Solid Edge part; units mm, degrees
sketch "Sketch1" plane through (0, 0, 0) normal (0, -1, 0) x (1, 0, 0)
  line L0 (0, 21.7) -> (4.505, 21.7)
  line L1 (4.505, 21.7) -> (4.505, 18.25)
  line L2 (4.505, 18.25) -> (2.1, 18.25)
  line L3 (2.1, 18.25) -> (2.1, 17.85)
  line L4 (2.1, 17.85) -> (2.5, 17.85)
  line L5 (2.5, 17.85) -> (2.5, 7.25)
  line L6 (2.5, 7.25) -> (2, 7.25)
  line L7 (2, 7.25) -> (2, 0)
  line L8 (2, 0) -> (0, 0)
  dimension "D1" = 4.505
  dimension "D2" = 2.1
  dimension "D3" = 2
  dimension "D4" = 2.5
  dimension "D5" = 2
revolve "RevolvedProtrusion1" add sketch "Sketch1" angle 360 about axis through (0, 0, 0) along (0, 0, 1)
chamfer "Chamfer1" distance 0.3 angle 45 3 edges at (-2.5, 0, 17.85) (-4.505, 0, 21.7) (-2, 0, 0)
fillet "Round_1" radius 0.2 4 edges at (-4.505, 0, 18.25) (-2.1, 0, 18.25) (-2.5, 0, 7.25) (-2.5, 0, 17.55)
sketch "Sketch2" plane through (0, 0, 21.7) normal (0, 0, 1) x (1, 0, 0)
  line L0 (1.5, 0.866) -> (0, 1.7321)
  line L1 (0, 1.7321) -> (-1.5, 0.866)
  line L2 (-1.5, 0.866) -> (-1.5, -0.866)
  line L3 (-1.5, -0.866) -> (0, -1.7321)
  line L4 (0, -1.7321) -> (1.5, -0.866)
  line L5 (1.5, -0.866) -> (1.5, 0.866)
extrude "ExtrudedCutout_1" cut sketch "Sketch2" against normal blind 2.4
properties material "Stainless Steel, 304"
Verification items for the finished model (mm, model axes). A direction names the side the tool comes from. Coordinates: 2 decimals unless noted, no trailing zeros. Order: outer loops, then holes, each group sorted by start corner. A loop starts at its lowest first (then second) coordinate and runs counter-clockwise, first axis right, second up. Notation, with made-up numbers: (-17, 18.25) -> (17, 18.25) arc R31 cw to (17, 51.25) -> close; hole circle Ø10 at (-3.5, 26). An arc over 180 degrees is marked (long way). Put each result on its own line as item: value. Start each with the question number.
1. Access from +Z, -Z, +X, -X, +Y, -Y to the whole of each face (thin tool, end or side, straight path). Record for faces 5 (the flat face through (0.74, -1.305, 20.517)), 6 (the flat face through (0, 0, 0)), 7 (the cylindrical face through (0, 2, 4)).
2. Go/stop test with flat-tipped pins: pin 1 Ø1 at (y, z) = (2.5, 13) entering from -X; pin 2 Ø2 at (y, z) = (0.5, 10.5) entering from -X; pin 3 Ø1.5 at (y, z) = (-0.5, 12.5) entering from +X. Record where each tip stops, or that it passes through.
3. Cross-section at B-B, the plane z = 4.5. Record the boundary of the cut face in (x, y).
4. Cross-section at A-A, the plane z = 8.75. Record the boundary of the cut face in (x, y), then the cut area to 3 significant figures.
5. Material ranges on L1, parallel to X at y = 2, z = 9.25; L2, parallel to Z at x = 3.75, y = -0.25; L3, parallel to Y at x = -1, z = 1.5, recorded low to high. Write a range as [from, to].
6. Mould release check, pull along Y, two halves, no side actions. Record for faces 1 (the flat face through (2, 0, 21.7)), 2 (the cylindrical face through (4.3, -1.35, 19.9)), 3 (the flat face through (0, 0, 19.3)), 4 (the flat face through (-0.74, 1.305, 20.517)): released by +Y, released by -Y, zero draft, split by the parting line, or undercut.
Computed:
1. face 5: +Z
1. face 6: -Z, +X, -X, +Y, -Y
1. face 7: -Z
2. pin 1: x = -1.5
2. pin 2: x = -2.5
2. pin 3: x = 2.5
3. outline: circle Ø4 at (0, 0)
4. outline: circle Ø5 at (0, 0)
4. area: 19.6 mm2
5. L1: [-1.5, 1.5]
5. L2: [18.25, 21.7]
5. L3: [-1.73, 1.73]
6. face 1: zero draft
6. face 2: split by the parting line
6. face 3: undercut
6. face 4: undercut
